CAD build for the part. Positions are in the model's coordinates, mm. A direction names the side the tool comes from. Give positions to 0.01 mm unless a question says otherwise; leave off trailing zeros. Loops run counter-clockwise (first coordinate to the right, second up) from the corner with the lowest first, then second, coordinate; pieces in that order, holes last. Notation, with made-up numbers: M 42.25,-22.5 L 49.25,-22.5 A22 ccw 49.25,3.5 Z; hole C -28,-8 d7. An arc over 180 degrees is marked long. One line per question, with ' | ' between items.
```python
from build123d import *

# Parameters (mm, degrees)
BOSS_EXTRUDE1_DEPTH = 12.7
CUT_EXTRUDE1_REACH  = 188.026
SKETCH2_R           = 2.5
SKETCH2_R_2         = 17.78
SKETCH2_R_3         = 11
SKETCH2_R_4         = 1.7


with BuildPart() as part:
    # Sketch1 → Boss-Extrude1 (new body)
    with BuildSketch(Plane(origin=(0, 0, 0), x_dir=(1, 0, 0), z_dir=(0, 1, 0))):
        Polygon((151.7015, 53.213), (151.7015, 51.7525), (176.3395, 51.7525), (176.3395, 27.1145), (177.8, 27.1145), (177.8, -27.1145), (176.3395, -27.1145), (176.3395, -51.7525), (151.7015, -51.7525), (151.7015, -53.213), (-151.7015, -53.213), (-151.7015, -51.7525), (-176.3395, -51.7525), (-176.3395, -27.1145), (-177.8, -27.1145), (-177.8, 27.1145), (-176.3395, 27.1145), (-176.3395, 51.7525), (-151.7015, 51.7525), (-151.7015, 53.213), align=None)
    extrude(amount=BOSS_EXTRUDE1_DEPTH)

    # Sketch2 → Cut-Extrude1 (cut, up to next)
    with BuildSketch(Plane(origin=(0, 12.7, 0), x_dir=(1, 0, 0), z_dir=(0, 1, 0)), mode=Mode.PRIVATE) as cut_extrude1_sk1:
        with Locations(Location((133.3, -28, 0), (0, 0, 270))):
            Circle(SKETCH2_R)
    cut_extrude1_tool1 = extrude(cut_extrude1_sk1.sketch, amount=-CUT_EXTRUDE1_REACH, mode=Mode.PRIVATE) & part.part
    # Sketch2 → Cut-Extrude1 (cut, up to next)
    with BuildSketch(Plane(origin=(0, 12.7, 0), x_dir=(1, 0, 0), z_dir=(0, 1, 0)), mode=Mode.PRIVATE) as cut_extrude1_sk2:
        with Locations(Location((77.3, -28, 0), (0, 0, 90))):
            Circle(SKETCH2_R)
    cut_extrude1_tool2 = extrude(cut_extrude1_sk2.sketch, amount=-CUT_EXTRUDE1_REACH, mode=Mode.PRIVATE) & part.part
    # Sketch2 → Cut-Extrude1 (cut, up to next)
    with BuildSketch(Plane(origin=(0, 12.7, 0), x_dir=(1, 0, 0), z_dir=(0, 1, 0)), mode=Mode.PRIVATE) as cut_extrude1_sk3:
        with Locations(Location((133.3, 28, 0), (0, 0, 90))):
            Circle(SKETCH2_R)
    cut_extrude1_tool3 = extrude(cut_extrude1_sk3.sketch, amount=-CUT_EXTRUDE1_REACH, mode=Mode.PRIVATE) & part.part
    # Sketch2 → Cut-Extrude1 (cut, up to next)
    with BuildSketch(Plane(origin=(0, 12.7, 0), x_dir=(1, 0, 0), z_dir=(0, 1, 0)), mode=Mode.PRIVATE) as cut_extrude1_sk4:
        with Locations(Location((77.3, 28, 0), (0, 0, 270))):
            Circle(SKETCH2_R)
    cut_extrude1_tool4 = extrude(cut_extrude1_sk4.sketch, amount=-CUT_EXTRUDE1_REACH, mode=Mode.PRIVATE) & part.part
    # Sketch2 → Cut-Extrude1 (cut, up to next)
    with BuildSketch(Plane(origin=(0, 12.7, 0), x_dir=(1, 0, 0), z_dir=(0, 1, 0)), mode=Mode.PRIVATE) as cut_extrude1_sk5:
        with Locations(Location((105.3, 0, 0), (0, 0, 270))):
            Circle(SKETCH2_R_2)
    cut_extrude1_tool5 = extrude(cut_extrude1_sk5.sketch, amount=-CUT_EXTRUDE1_REACH, mode=Mode.PRIVATE) & part.part
    # Sketch2 → Cut-Extrude1 (cut, up to next)
    with BuildSketch(Plane(origin=(0, 12.7, 0), x_dir=(1, 0, 0), z_dir=(0, 1, 0)), mode=Mode.PRIVATE) as cut_extrude1_sk6:
        with Locations(Location((-85.2, 0, 0), (0, 0, 270))):
            Circle(SKETCH2_R_3)
    cut_extrude1_tool6 = extrude(cut_extrude1_sk6.sketch, amount=-CUT_EXTRUDE1_REACH, mode=Mode.PRIVATE) & part.part
    # Sketch2 → Cut-Extrude1 (cut, up to next)
    with BuildSketch(Plane(origin=(0, 12.7, 0), x_dir=(1, 0, 0), z_dir=(0, 1, 0)), mode=Mode.PRIVATE) as cut_extrude1_sk7:
        with Locations(Location((-100.7, 15.5, 0), (0, 0, 270))):
            Circle(SKETCH2_R_4)
    cut_extrude1_tool7 = extrude(cut_extrude1_sk7.sketch, amount=-CUT_EXTRUDE1_REACH, mode=Mode.PRIVATE) & part.part
    # Sketch2 → Cut-Extrude1 (cut, up to next)
    with BuildSketch(Plane(origin=(0, 12.7, 0), x_dir=(1, 0, 0), z_dir=(0, 1, 0)), mode=Mode.PRIVATE) as cut_extrude1_sk8:
        with Locations(Location((-69.7, 15.5, 0), (0, 0, 90))):
            Circle(SKETCH2_R_4)
    cut_extrude1_tool8 = extrude(cut_extrude1_sk8.sketch, amount=-CUT_EXTRUDE1_REACH, mode=Mode.PRIVATE) & part.part
    # Sketch2 → Cut-Extrude1 (cut, up to next)
    with BuildSketch(Plane(origin=(0, 12.7, 0), x_dir=(1, 0, 0), z_dir=(0, 1, 0)), mode=Mode.PRIVATE) as cut_extrude1_sk9:
        with Locations(Location((-69.7, -15.5, 0), (0, 0, 270))):
            Circle(SKETCH2_R_4)
    cut_extrude1_tool9 = extrude(cut_extrude1_sk9.sketch, amount=-CUT_EXTRUDE1_REACH, mode=Mode.PRIVATE) & part.part
    # Sketch2 → Cut-Extrude1 (cut, up to next)
    with BuildSketch(Plane(origin=(0, 12.7, 0), x_dir=(1, 0, 0), z_dir=(0, 1, 0)), mode=Mode.PRIVATE) as cut_extrude1_sk10:
        with Locations(Location((-100.7, -15.5, 0), (0, 0, 90))):
            Circle(SKETCH2_R_4)
    cut_extrude1_tool10 = extrude(cut_extrude1_sk10.sketch, amount=-CUT_EXTRUDE1_REACH, mode=Mode.PRIVATE) & part.part
    add(cut_extrude1_tool1.solids().sort_by_distance((133.3, 12.7, 28))[0], mode=Mode.SUBTRACT)
    add(cut_extrude1_tool2.solids().sort_by_distance((77.3, 12.7, 28))[0], mode=Mode.SUBTRACT)
    add(cut_extrude1_tool3.solids().sort_by_distance((133.3, 12.7, -28))[0], mode=Mode.SUBTRACT)
    add(cut_extrude1_tool4.solids().sort_by_distance((77.3, 12.7, -28))[0], mode=Mode.SUBTRACT)
    add(cut_extrude1_tool5.solids().sort_by_distance((105.3, 12.7, 0))[0], mode=Mode.SUBTRACT)
    add(cut_extrude1_tool6.solids().sort_by_distance((-85.2, 12.7, 0))[0], mode=Mode.SUBTRACT)
    add(cut_extrude1_tool7.solids().sort_by_distance((-100.7, 12.7, -15.5))[0], mode=Mode.SUBTRACT)
    add(cut_extrude1_tool8.solids().sort_by_distance((-69.7, 12.7, -15.5))[0], mode=Mode.SUBTRACT)
    add(cut_extrude1_tool9.solids().sort_by_distance((-69.7, 12.7, 15.5))[0], mode=Mode.SUBTRACT)
    add(cut_extrude1_tool10.solids().sort_by_distance((-100.7, 12.7, 15.5))[0], mode=Mode.SUBTRACT)


solid = part.part
```
Item 1: Saw through at C-C on z = 0. Give the cut face in (x, y), and give its area (3 significant figures).
Conclusion:
outline: M -177.8,0 L -96.2,0 L -96.2,12.7 L -177.8,12.7 Z; M -74.2,0 L 87.52,0 L 87.52,12.7 L -74.2,12.7 Z; M 123.08,0 L 177.8,0 L 177.8,12.7 L 123.08,12.7 Z | area: 3,790 mm²
Item 2: Drill centre lines: line 1 along X through (y, z) = (1.5, 0); line 2 along Z through (x, y) = (-100.5, 4); line 3 along X through (y, z) = (9.75, -28). Where is each one in solid material? Low to high. Write a range as [from, to].
Conclusion:
line 1: [-177.8, -96.2], [-74.2, 87.52], [123.08, 177.8] | line 2: [-53.21, -17.19], [-13.81, 13.81], [17.19, 53.21] | line 3: [-176.34, 74.8], [79.8, 130.8], [135.8, 176.34]
Item 3: Mould opens along Z. For faces 4 (the flat face through (177.8, 6, 0)), 5 (the cylindrical face through (87.94, 6.44, -3.85)), 6 (the flat face through (-164, 6, -51.752)) say: pulls with the +Z half, pulls with the -Z half, needs draft (parallel to the pull), parting line crosses it, or undercut.
Conclusion:
face 4: needs draft | face 5: undercut | face 6: pulls with the -Z half
Item 4: 3-axis set-ups, long thin cutter, end or side, ignore diameter. For faces 1 (the flat face through (-164, 6, 51.752)), 2 (the flat face through (176.34, 6, -40)), 3 (the flat face through (176.34, 6, 39)): which of +Z, -Z, +X, -X, +Y, -Y reach the whole face in a straight line?
Conclusion:
face 1: +Z, -X, +Y, -Y | face 2: -Z, +X, +Y, -Y | face 3: +Z, +X, +Y, -Y
Item 5: Saw through at A-A on x = -85.2. Give the cut face in (y, z), and give its area (3 significant figures).
Conclusion:
outline: M 0,-53.21 L 12.7,-53.21 L 12.7,-11 L 0,-11 Z; M 0,11 L 12.7,11 L 12.7,53.21 L 0,53.21 Z | area: 1,070 mm²
Item 6: Drop flat-ended pins along their axis: P1, Ø3, axis at x = 77.3, z = -28, coming from the -Y side; P2, Ø0.7, axis at y = 7, z = -52.5, coming from the +X side; P3, Ø6.5, axis at y = 9.5, z = -44.5, coming from the -X side; P4, Ø0.7, axis at x = 177.5, y = 7, coming from the -Z side. Give the stop position or say it passes through.
Conclusion:
P1: through | P2: x = 151.7 | P3: x = -176.34 | P4: z = -27.11
Item 7: Saw through at B-B on y = 7.25. State how many separate pieces and enclosed holes the cut face has, and give its area (3 significant figures).
Conclusion:
separate pieces: 1 | enclosed holes: 10 | area: 36,100 mm²
